The listing builds one solid part. Answer for the finished solid, in the listing's coordinates (mm). Face numbers are marked on the shaded views. A direction names the side the tool comes from. Coordinates: 2 decimals unless noted, no trailing zeros. Order: outer loops, then holes, each group sorted by start corner. A loop starts at its lowest first (then second) coordinate and runs counter-clockwise, first axis right, second up. Notation, with made-up numbers: (25, 78) -> (34, 78) arc R20 cw to (34, 94) -> close; hole circle Ø8 at (81.25, 52.25). An arc over 180 degrees is marked (long way). Return JSON: item names as keys, results as strings.
Autodesk Inventor part; units mm, degrees
ref_plane "YZ Plane" through (0, 0, 0) normal (1, 0, 0) x (0, 1, 0)
ref_plane "XZ Plane" through (0, 0, 0) normal (0, 1, 0) x (-1, 0, 0)
ref_plane "XY Plane" through (0, 0, 0) normal (0, 0, 1) x (1, 0, 0)
sketch "Sketch1" plane through (0, 0, 0) normal (1, 0, 0) x (0, 1, 0)
  circle A0 centre (0, 0) radius 7.45
  dimension "d0" = 14.9
extrude "Extrusion1" add sketch "Sketch1" along normal blind 70
sketch "Sketch2" plane through (70, 0, 0) normal (1, 0, 0) x (0, 0, -1)
  line L0 (0, 14.962) -> (12.9575, 7.481)
  line L1 (12.9575, 7.481) -> (12.9575, -7.481)
  line L2 (12.9575, -7.481) -> (0, -14.962)
  line L3 (0, -14.962) -> (-12.9575, -7.481)
  line L4 (-12.9575, -7.481) -> (-12.9575, 7.481)
  line L5 (-12.9575, 7.481) -> (0, 14.962)
  point P0 (0, 0)
  point P1 (0, 0)
  dimension "d12" = 25.915
  dimension "d13" = 14.962
extrude "Extrusion2" add sketch "Sketch2" along normal blind 7
chamfer "Chamfer1" distance 1 angle 45 1 edges at (0, -7.45, 0)
sketch "Sketch3" plane through (0, 0, 0) normal (0, 0, 1) x (1, 0, 0)
  point P0 (0, 0)
thread "Thread2"
chamfer "Chamfer2" distance 2 angle 45 6 edges at (77, 11.2215, -6.4788) (77, 11.2215, 6.4788) (77, 0, 12.9575) (77, -11.2215, 6.4788) (77, -11.2215, -6.4788) (77, 0, -12.9575)
properties part number "bolt" material "Iron, Cast"
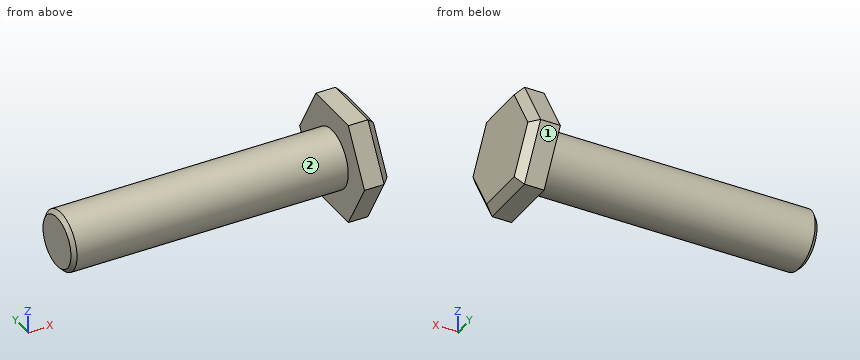
1. The part is cut by section D-D on y = 8.5. Give the vertices of the cut face in (x, z).
Answer block:
{"outline": "(70, -11.19) -> (75, -11.19) -> (77, -7.19) -> (77, 7.19) -> (75, 11.19) -> (70, 11.19) -> close"}
2. For the marked faces 1 and 2, determine the directions among +Z, -Z, +X, -X, +Y, -Y from which every point of the face is accessible in a straight line to the end or side of a thin tool.
Answer block:
{"face 1": "-Z, +X, -X, +Y", "face 2": "-X"}
3. The part is cut by section A-A on x = 71. Give the vertices of the cut face in (y, z).
Answer block:
{"outline": "(-14.96, 0) -> (-7.48, -12.96) -> (7.48, -12.96) -> (14.96, 0) -> (7.48, 12.96) -> (-7.48, 12.96) -> close"}
4. Consider line 1 (X direction, y = 10.5, z = 1.75); line 2 (Y direction, x = 16.5, z = 0.25); line 3 (Z direction, x = 6, y = 6.5). Determine where each line is inside the solid, lowest interval first. Write a range as from..to.
Answer block:
{"line 1": "x = 70..77", "line 2": "y = -7.45..7.45", "line 3": "z = -3.64..3.64"}
5. The part is cut by section B-B on y = 0. Give the vertices of the cut face in (x, z), and give its area (3 significant figures).
Answer block:
{"outline": "(0, -6.45) -> (1, -7.45) -> (70, -7.45) -> (70, -12.96) -> (75, -12.96) -> (77, -10.96) -> (77, 10.96) -> (75, 12.96) -> (70, 12.96) -> (70, 7.45) -> (1, 7.45) -> (0, 6.45) -> close", "area": "1,220 mm2"}
6. Each of these flat-tipped pins is pushed along its axis until it touches: pin 1 Ø10 at (x, y) = (47, -7) entering from -Z; pin 2 Ø8 at (x, y) = (50.5, 1) entering from +Z; pin 3 Ø5 at (x, y) = (11.5, 4.5) entering from +Z. Where does it stop, or does it pass through?
Answer block:
{"pin 1": "stops at z = -7.18", "pin 2": "stops at z = 7.45", "pin 3": "stops at z = 7.18"}
7. The part is cut by section C-C on x = 5. Give the vertices of the cut face in (y, z), and give its area (3 significant figures).
Answer block:
{"outline": "circle Ø14.9 at (0, 0)", "area": "174 mm2"}
